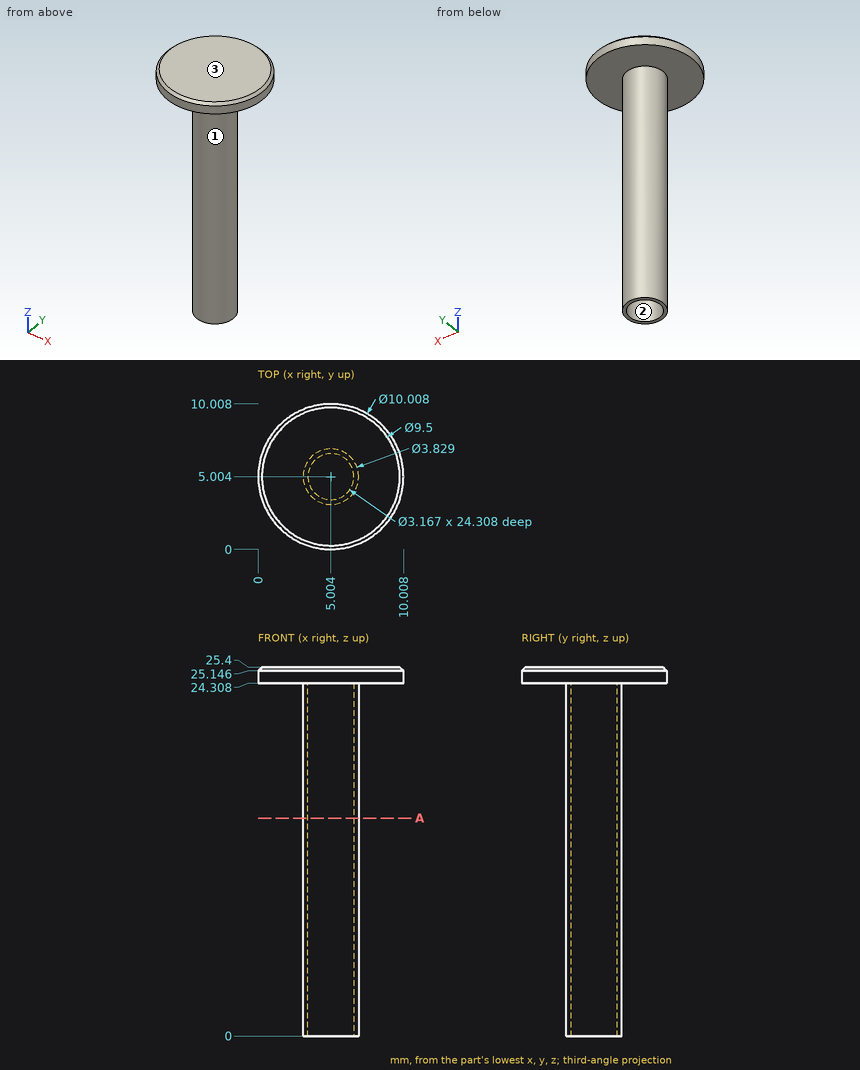
The figure shows three views and two pictorial views of one solid part (mm, origin at its lowest corner). Answer the questions. Round coordinates to 2 decimals unless told otherwise and drop trailing zeros. Order: outer loops, then holes, each group sorted by start corner. A loop starts at its lowest first (then second) coordinate and runs counter-clockwise, first axis right, second up. Notation, with made-up numbers: M 3.25,73 L 62.25,73 A32 cw 62.25,111 Z; hole C 11.25,-33 d4. An arc over 180 degrees is marked long. Put each result on its own line as item: value. Start each with the question number.
Q1. For a pull along X with two mould halves and no side action, classify the marked faces 1, 2 and 3 as pulls with the +X half, pulls with the -X half, needs draft (parallel to the pull), parting line crosses it, or undercut.
Q2. Section A-A, the plane z = 15 is taken. Write down the section's boundary in (x, y) (1 decimal).
Q3. Straight lines are drawn through the part: L1, parallel to Z at x = 4, y = 9.25; L2, parallel to X at y = 5, z = 9.75; L3, parallel to X at y = 4.25, z = 17.5 (1 decimal). For each, find the intervals that lie inside material, in ascending order. Write a range as [from, to].
Q4. Flat-ended cylindrical pins translate along their axes: pin 1 (5 mm diameter, centred on x = 7, z = 4, fed in from +Y); pin 2 (1 mm diameter, centred on y = 8.5, z = 11, fed in from +X); pin 3 (2 mm diameter, centred on x = 3, z = 17.5, fed in from -Y); pin 4 (6 mm diameter, centred on y = 2.5, z = 20, fed in from +X). Find the tip coordinate at first contact, or state that the pin passes through.
Findings below:
1. face 1: parting line crosses it
1. face 2: undercut
1. face 3: needs draft
2. outline: C 5,5 d3.8; hole C 5,5 d3.2
3. L1: z = [24.31, 25.4]
3. L2: x = [3.09, 3.42], [6.59, 6.92]
3. L3: x = [3.2, 3.6], [6.4, 6.8]
4. pin 1: stops at y = 6.92
4. pin 2: passes through
4. pin 3: stops at y = 3.37
4. pin 4: stops at x = 6.92
